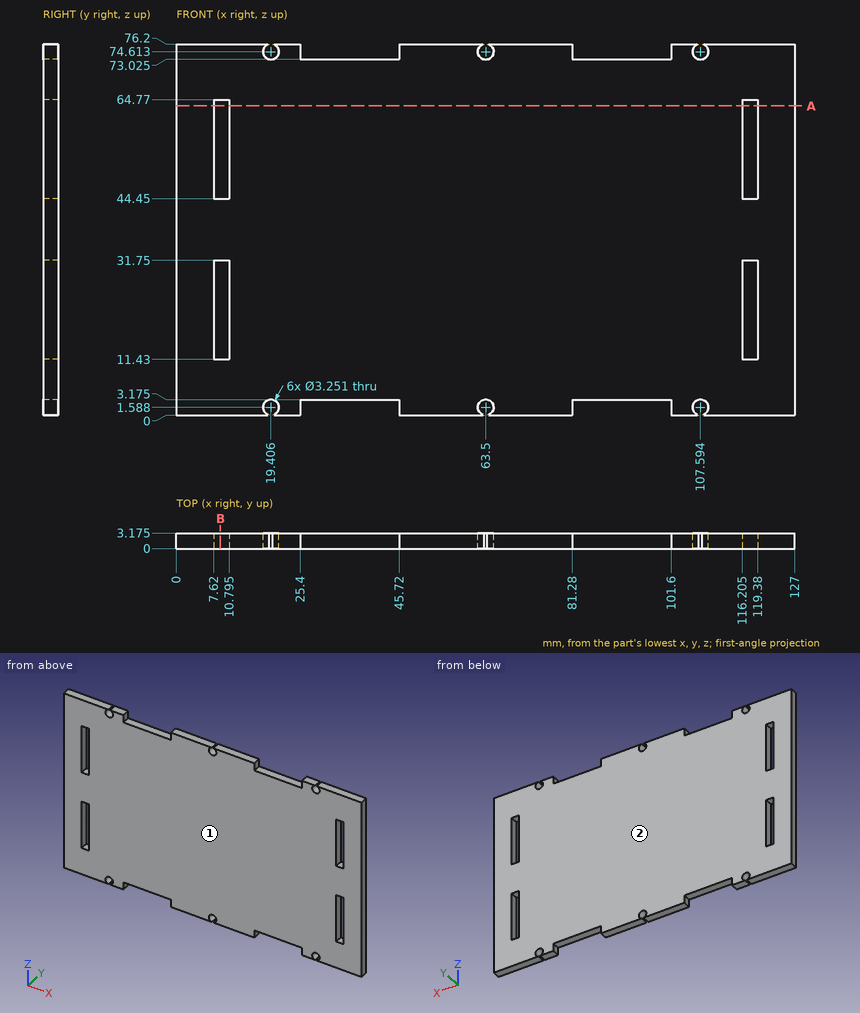
Answer from the drawing. Dimensions are ordinates in mm from the lowest x, y and z of the part. Give positions to 0.01 mm unless a question says otherwise; leave off trailing zeros. Loops run counter-clockwise (first coordinate to the right, second up) from the corner with the lowest first, then second, coordinate; pieces in that order, holes last. Notation, with made-up numbers: M 45,-26 L 58,-26 A11 cw 58,-22 Z; hole C 33.5,67 d5. An arc over 180 degrees is marked long. One line per item, written item: value.
Q1. A cutting plane is placed at A-A on z = 63.5. Determine the outline of the cut face in (x, y) (1 decimal).
Working result:
outline: M 0,0 L 7.6,0 L 7.6,3.2 L 0,3.2 Z; M 10.8,0 L 116.2,0 L 116.2,3.2 L 10.8,3.2 Z; M 119.4,0 L 127,0 L 127,3.2 L 119.4,3.2 Z
Q2. Determine the mould class of the marked faces 1 and 2 for opening direction Y: +Y half, -Y half, draft (parallel to the pull), parting line (faces both ways), or undercut.
Working result:
face 1: -Y half
face 2: +Y half
Q3. A cutting plane is placed at B-B on x = 9. Give the number of separate pieces and of enclosed holes in the cut face, then the cut area to 3 significant figures.
Working result:
separate pieces: 3
enclosed holes: 0
area: 113 mm^2
Q4. Find the intervals of material crossed by line 1 (X direction, y = 1.8, z = 28) (1 decimal); line 2 (Z direction, x = 98, y = 1.6) (1 decimal), in increasing order. Write a range as from..to.
Working result:
line 1: x = 0..7.6, 10.8..116.2, 119.4..127
line 2: z = 3.2..73
Q5. Flat-ended cylindrical pins translate along their axes: P1, Ø1, axis at y = 1.5, z = 75, coming from the -X side; P2, Ø1, axis at x = 44.5, y = 1.5, coming from the -Z side (1 decimal). Find the tip coordinate at first contact, or state that the pin passes through.
Working result:
P1: stops at x = 0
P2: stops at z = 3.2
